```python
from build123d import *

# Parameters (mm, degrees)
SKETCH1_R           = 7.05
SKETCH1_R_2         = 4.05
BOSS_EXTRUDE1_DEPTH = 160
SKETCH3_W           = 15
SKETCH3_H           = 15
BOSS_EXTRUDE2_DEPTH = 10
BOSS_EXTRUDE3_DEPTH = 20
CIRPATTERN1_COUNT   = 2
FILLET1_R           = 10
CUT_EXTRUDE2_DEPTH  = 40
SKETCH6_R           = 2
CUT_EXTRUDE3_DEPTH  = 173.37314178
SKETCH7_R           = 3.75
CUT_EXTRUDE4_DEPTH  = 4


with BuildPart() as part:
    # Sketch1 → Boss-Extrude1 (new body)
    # profile 1 of 2: a face of its own
    with BuildSketch(Plane.XY):
        Circle(SKETCH1_R)
        Circle(SKETCH1_R_2, mode=Mode.SUBTRACT)
    # profile 2 of 2: a face of its own
    with BuildSketch(Plane.XY):
        Circle(SKETCH1_R_2)
    extrude(amount=BOSS_EXTRUDE1_DEPTH)

    # Sketch3 → Boss-Extrude2 (add)
    with BuildSketch(Plane(origin=(0, 0, 0), x_dir=(-1, 0, 0), z_dir=(0, 0, -1))):
        Rectangle(SKETCH3_W, SKETCH3_H)
    extrude(amount=BOSS_EXTRUDE2_DEPTH)

    # Sketch4 → Boss-Extrude3 (add)
    with BuildSketch(Plane(origin=(0, 7.5, 0), x_dir=(1, 0, 0), z_dir=(0, 1, 0))):
        Polygon((-0.386751346, 10), (5.386751346, 0), (0.386751346, 0), (-5.386751346, 10), align=None)
    boss_extrude3 = extrude(amount=BOSS_EXTRUDE3_DEPTH)

    # CirPattern1: Boss-Extrude3 ×2 about axis
    cirpattern1_axis = Axis((0, 0, 0), (0, 0, 1))
    for i in range(1, CIRPATTERN1_COUNT):
        add(boss_extrude3.rotate(cirpattern1_axis, i * 360 / CIRPATTERN1_COUNT))

    # Fillet1
    # the kernel refuses this fillet: 10 mm, written as the material it adds along each edge
    with BuildSketch(Plane(origin=(0, 0, 0), x_dir=(1, 0, 0), z_dir=(0, -1, 0))) as fillet1_piece_1_section:
        with BuildLine():
            CenterArc((7.05 + FILLET1_R, FILLET1_R), FILLET1_R, 180, 90)
            Line((7.05, FILLET1_R), (7.05, 0))
            Line((7.05, 0), (7.05 + FILLET1_R, 0))
        make_face()
    fillet1_piece_1 = revolve(axis=Axis((0, 0, 0), (0, 0, 1)), mode=Mode.PRIVATE)
    fillet1_piece_1 = split(fillet1_piece_1, bisect_by=Plane(origin=(7.384958352, 7.5, 2.9516764), z_dir=(0, -1, 0)), keep=Keep.TOP, mode=Mode.PRIVATE)
    fillet1_piece_1 = split(fillet1_piece_1, bisect_by=Plane(origin=(7.5, 6.602416729, 2.9516764), z_dir=(-1, 0, 0)), keep=Keep.TOP, mode=Mode.PRIVATE)
    fillet1_piece_1 = split(fillet1_piece_1, bisect_by=Plane(origin=(-7.5, 6.602416729, 2.9516764), z_dir=(1, 0, 0)), keep=Keep.TOP, mode=Mode.PRIVATE)
    fillet1_piece_1 = split(fillet1_piece_1, bisect_by=Plane(origin=(7.384958352, -7.5, 2.9516764), z_dir=(0, 1, 0)), keep=Keep.TOP, mode=Mode.PRIVATE)
    add(fillet1_piece_1)
    with BuildSketch(Plane(origin=(0, 0, 0), x_dir=(1, 0, 0), z_dir=(0, -1, 0))) as fillet1_piece_2_section:
        with BuildLine():
            CenterArc((7.05 + FILLET1_R, FILLET1_R), FILLET1_R, 180, 90)
            Line((7.05, FILLET1_R), (7.05, 0))
            Line((7.05, 0), (7.05 + FILLET1_R, 0))
        make_face()
    fillet1_piece_2 = revolve(axis=Axis((0, 0, 0), (0, 0, 1)), mode=Mode.PRIVATE)
    fillet1_piece_2 = split(fillet1_piece_2, bisect_by=Plane(origin=(5.410380514, 9.830478865, 0.040926919), z_dir=(-0.8660254037844362, 0, 0.5000000000000043)), keep=Keep.TOP, mode=Mode.PRIVATE)
    fillet1_piece_2 = split(fillet1_piece_2, bisect_by=Plane(origin=(7.5, 9.830478865, 1.235681154), z_dir=(-1, 0, 0)), keep=Keep.TOP, mode=Mode.PRIVATE)
    fillet1_piece_2 = split(fillet1_piece_2, bisect_by=Plane(origin=(1.660380514, 9.830478865, 2.205990428), z_dir=(0.8660254037844359, 0, -0.5000000000000047)), keep=Keep.TOP, mode=Mode.PRIVATE)
    fillet1_piece_2 = split(fillet1_piece_2, bisect_by=Plane(origin=(3.341005476, -7.5, 1.235681154), z_dir=(0, 1, 0)), keep=Keep.TOP, mode=Mode.PRIVATE)
    add(fillet1_piece_2)
    with BuildSketch(Plane(origin=(0, 0, 0), x_dir=(1, 0, 0), z_dir=(0, -1, 0))) as fillet1_piece_3_section:
        with BuildLine():
            CenterArc((7.05 + FILLET1_R, FILLET1_R), FILLET1_R, 180, 90)
            Line((7.05, FILLET1_R), (7.05, 0))
            Line((7.05, 0), (7.05 + FILLET1_R, 0))
        make_face()
    fillet1_piece_3 = revolve(axis=Axis((0, 0, 0), (0, 0, 1)), mode=Mode.PRIVATE)
    fillet1_piece_3 = split(fillet1_piece_3, bisect_by=Plane(origin=(-3.341005467, -7.5, 1.235681156), z_dir=(0, -1, 0)), keep=Keep.TOP, mode=Mode.PRIVATE)
    fillet1_piece_3 = split(fillet1_piece_3, bisect_by=Plane(origin=(-5.410380512, -9.830478864, 0.040926917), z_dir=(0.8660254037844362, 0, 0.5000000000000043)), keep=Keep.TOP, mode=Mode.PRIVATE)
    fillet1_piece_3 = split(fillet1_piece_3, bisect_by=Plane(origin=(-1.660380512, -9.830478864, 2.205990426), z_dir=(-0.8660254037844359, 0, -0.5000000000000047)), keep=Keep.TOP, mode=Mode.PRIVATE)
    add(fillet1_piece_3)

    # Sketch5 → Cut-Extrude2 (cut)
    with BuildSketch(Plane.XY.offset(160)):
        with BuildLine():
            Line((2.664582519, 3.05), (-2.664582519, 3.05))
            ThreePointArc((-2.664582519, 3.05), (0, -4.05), (2.664582519, 3.05))
        make_face()
    extrude(amount=-CUT_EXTRUDE2_DEPTH, mode=Mode.SUBTRACT)

    # Sketch6 → Cut-Extrude3 (cut, through all)
    with BuildSketch(Plane(origin=(0, 0, -10), x_dir=(-1, 0, 0), z_dir=(0, 0, -1))):
        Circle(SKETCH6_R)
    extrude(amount=-CUT_EXTRUDE3_DEPTH, mode=Mode.SUBTRACT)

    # Sketch7 → Cut-Extrude4 (cut)
    with BuildSketch(Plane(origin=(0, 0, -10), x_dir=(-1, 0, 0), z_dir=(0, 0, -1))):
        Circle(SKETCH7_R)
    extrude(amount=-CUT_EXTRUDE4_DEPTH, mode=Mode.SUBTRACT)


solid = part.part
```
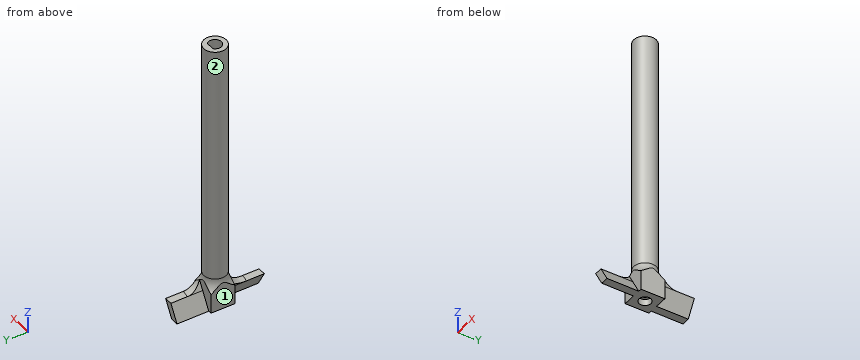
Can you work these out from the model? Positions are in its coordinate system, mm. Face numbers are marked on the shaded views. A direction names the side the tool comes from. Coordinates: 2 decimals unless noted, no trailing zeros. Loops run counter-clockwise (first coordinate to the right, second up) from the corner with the lowest first, then second, coordinate; pieces in that order, holes last. Notation, with made-up numbers: M 29,0.25 L 43,0.25 A14 cw 43,15.25 Z; hole C -15,49 d5. An arc over 180 degrees is marked long. Put each result on its own line as item: value. Start each with the question number.
(1) Which directions (+Z, -Z, +X, -X, +Y, -Y) give clear straight access to the entire face, cutting with the end or side of a thin tool? Please do the marked faces 1 and 2.
(2) Imagine slicing it at B-B on z = 104.5. List the corners of the cut face in (x, y) for me, and give its area (3 significant figures).
(3) Imagine slicing it at A-A on y = 0. List the corners of the cut face in (x, z) for me.
(4) Imagine slicing it at C-C on z = 136.5. List the corners of the cut face in (x, y) for me, and give its area (3 significant figures).
(5) I need wall thicknesses on probe 1 along Y at (x, z) = (0, 26); probe 2 along X at (y, z) = (0, 130.5); probe 3 along Y at (x, z) = (0, -8.8). Which ranges of each line are inside material? Lowest first, please.
(6) Will these pins go through, and if not, where does the flat tip stop? pin 1 Ø4 at (x, y) = (3.5, 19.5) entering from +Z; pin 2 Ø12 at (y, z) = (8.5, 19) entering from -X; pin 3 Ø3.5 at (x, y) = (1, -1) entering from +Z; pin 4 Ø2.5 at (x, y) = (0, 0) entering from +Z.
(7) Imagine slicing it at D-D on y = -21. List the corners of the cut face in (x, z) for me.
Worked answers:
1. face 1: +Z, -Z, -X, +Y, -Y
1. face 2: +Z
2. outline: C 0,0 d14.1; hole C 0,0 d4
2. area: 144 mm2
3. outline: M -7.5,-10 L -3.75,-10 L -3.75,-6 L -2,-6 L -2,120 L -4.05,120 L -4.05,160 L -7.05,160 L -7.05,10 A10 cw -7.5,7.03 Z; M 2,-6 L 3.75,-6 L 3.75,-10 L 7.5,-10 L 7.5,7.03 A10 cw 7.05,10 L 7.05,160 L 4.05,160 L 4.05,120 L 2,120 Z
4. outline: C 0,0 d14.1; hole M -2.66,3.05 A4.05 ccw long 2.66,3.05 Z
4. area: 108 mm2
5. probe 1: y = -7.05 to -2, 2 to 7.05
5. probe 2: x = -7.05 to -4.05, 4.05 to 7.05
5. probe 3: y = -27.5 to -3.75, 3.75 to 27.5
6. pin 1: stops at z = 0
6. pin 2: stops at x = -6.59
6. pin 3: stops at z = 120
6. pin 4: passes through
7. outline: M -5.39,0 L 0.39,-10 L 5.39,-10 L -0.39,0 Z
